Can you work these out from the model? Positions are in its coordinate system, mm. A direction names the side the tool comes from. Give positions to 0.01 mm unless a question says otherwise; leave off trailing zeros. Loops run counter-clockwise (first coordinate to the right, second up) from the corner with the lowest first, then second, coordinate; pieces in that order, holes last. Notation, with made-up numbers: M 23.5,27.25 L 38.5,27.25 A25 cw 38.5,55.25 Z; hole C 86.25,7 d3. An arc over 180 degrees is marked long. Use CSV: the item, a comma, the result in double quotes.
from build123d import *

# Parameters (mm, degrees)
SKETCH_1_W      = 12
SKETCH_1_H      = 10
SKETCH_1_R      = 0.8
EXTRUDE_1_DEPTH = 24
SKETCH_2_R      = 1.5
EXTRUDE_2_DEPTH = 9.3


with BuildPart() as part:
    # 스케치1 → 보스-돌출1 (new body)
    with BuildSketch(Plane(origin=(0, 0, 0), x_dir=(1, 0, 0), z_dir=(0, 1, 0))):
        Rectangle(SKETCH_1_W, SKETCH_1_H)
        with Locations(Location((4.5, 0, 0), (0, 0, 270))):
            Circle(SKETCH_1_R, mode=Mode.SUBTRACT)
        with Locations(Location((-4.5, 0, 0), (0, 0, 270))):
            Circle(SKETCH_1_R, mode=Mode.SUBTRACT)
    extrude(amount=EXTRUDE_1_DEPTH)

    # 스케치2 → 보스-돌출2 (add)
    with BuildSketch(Plane(origin=(0, 24, 0), x_dir=(1, 0, 0), z_dir=(0, 1, 0))):
        with Locations(Location((0, 0, 0), (0, 0, 90))):
            Circle(SKETCH_2_R)
    extrude(amount=EXTRUDE_2_DEPTH)


solid = part.part
Q1. I'm going to push a flat-ended pin straight in: P1, Ø1.8, axis at x = 4.5, z = 0, coming from the +Y side. Where does the tip first touch, or does it pass through?
Model answer:
P1,"y = 24"
Q2. For faces 4 (the flat face through (-1.4, 24, -1.2)), 5 (the cylindrical face through (3.72, 11.83, -0.17)), which set-ups out of +Z, -Z, +X, -X, +Y, -Y let a thin tool reach every point of the face, with its end or its side?
Model answer:
face 4,"+Y"
face 5,"+Y, -Y"
Q3. Please list where these lines run through material, in increasing order: L1, parallel to X at y = 17.25, z = 0; L2, parallel to Y at x = -3.5, z = -0.5; L3, parallel to Z at x = 4.25, y = 10.5. Write a range as from..to.
Model answer:
L1,"-6..-5.3, -3.7..3.7, 5.3..6"
L2,"0..24"
L3,"-5..-0.76, 0.76..5"
Q4. If we mould it in two halves opening along X, with no side actions, what happens to faces 1 (the flat face through (6, 12, 0)), 2 (the cylindrical face through (-5.28, 11.83, -0.17)), 3 (the flat face through (0, 12, 5))? For each: released by +X, released by -X, zero draft, split by the parting line, or undercut.
Model answer:
face 1,"released by +X"
face 2,"undercut"
face 3,"zero draft"
Q5. I want a section at C-C, the plane y = 2.5. Please give me the cut outline in (x, z).
Model answer:
outline,"M -6,-5 L 6,-5 L 6,5 L -6,5 Z; hole C -4.5,0 d1.6; hole C 4.5,0 d1.6"
Q6. I want a section at B-B, the plane x = 4.5. Please give me the cut outline in (y, z).
Model answer:
outline,"M 0,-5 L 24,-5 L 24,-0.8 L 0,-0.8 Z; M 0,0.8 L 24,0.8 L 24,5 L 0,5 Z"
Q7. I want a section at A-A, the plane z = 0. Please give me the cut outline in (x, y), then the cut area to 3 significant figures.
Model answer:
outline,"M -6,0 L -5.3,0 L -5.3,24 L -6,24 Z; M -3.7,0 L 3.7,0 L 3.7,24 L 1.5,24 L 1.5,33.3 L -1.5,33.3 L -1.5,24 L -3.7,24 Z; M 5.3,0 L 6,0 L 6,24 L 5.3,24 Z"
area,"239 mm2"
Q8. I want a section at D-D, the plane x = 0. Please give me the cut outline in (y, z), then the cut area to 3 significant figures.
Model answer:
outline,"M 0,-5 L 24,-5 L 24,-1.5 L 33.3,-1.5 L 33.3,1.5 L 24,1.5 L 24,5 L 0,5 Z"
area,"268 mm2"
